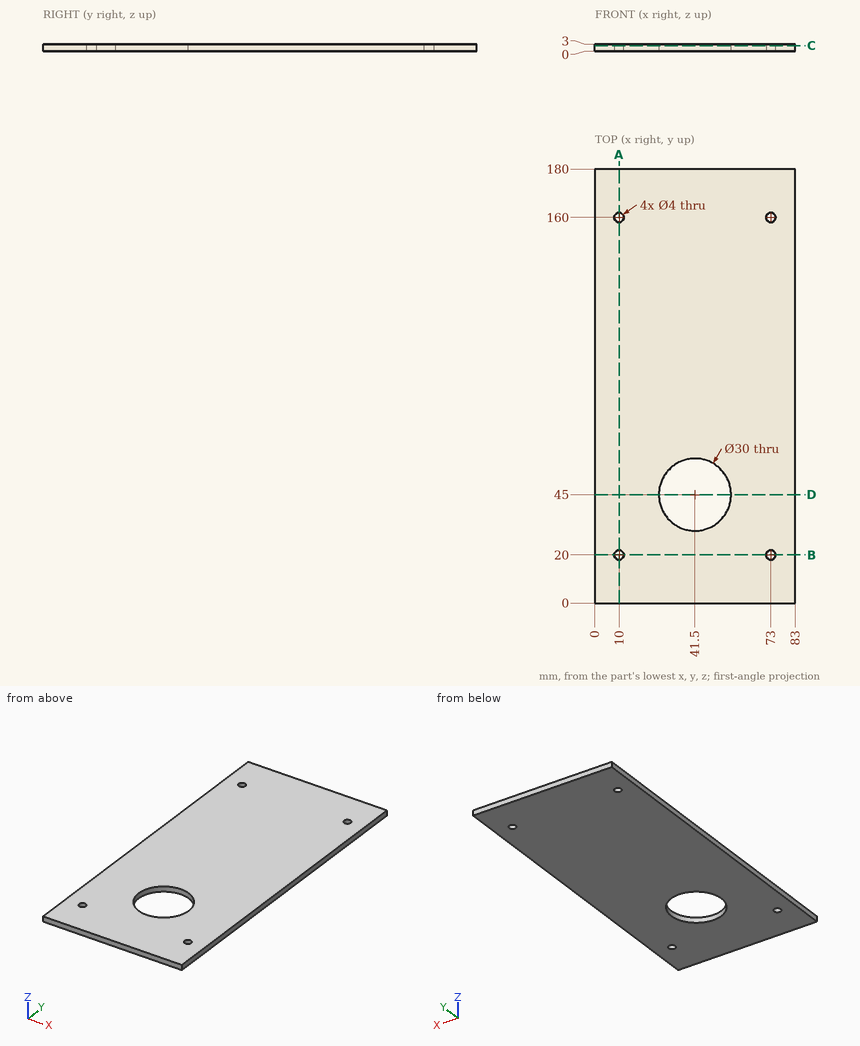
For this review, use the dimensioned drawing (mm, ordinates from the lowest corner) and the shaded views. Coordinates: 2 decimals unless noted, no trailing zeros. Loops run counter-clockwise (first coordinate to the right, second up) from the corner with the lowest first, then second, coordinate; pieces in that order, holes last. Notation, with made-up numbers: (35, 21) -> (80, 21) arc R26 ccw to (80, 50) -> close; hole circle Ø6 at (-24, 22). An arc over 180 degrees is marked (long way). Use a Markdown table: item, result. Add a question column.
1. Add section A-A on x = 10. Write out the cut boundary in (y, z).
2. Add section D-D on y = 45. Write out the cut boundary in (x, z).
3. Add section B-B on y = 20. Write out the cut boundary in (x, z), plus the area to 3 significant figures.
4. Add section C-C on z = 2.3. Write out the cut boundary in (x, y).
5. To check wall thickness, follow line 1 (X direction, y = 20, z = 0.8); line 2 (Y direction, x = 73, z = 2.1); line 3 (Y direction, x = 41.5, z = 0.85). State the ranges of each line that lie inside material, in increasing order.
Returned:
| question | item | result |
|---|---|---|
| 1 | outline | (0, 0) -> (18, 0) -> (18, 3) -> (0, 3) -> close; (22, 0) -> (158, 0) -> (158, 3) -> (22, 3) -> close; (162, 0) -> (180, 0) -> (180, 3) -> (162, 3) -> close |
| 2 | outline | (0, 0) -> (26.5, 0) -> (26.5, 3) -> (0, 3) -> close; (56.5, 0) -> (83, 0) -> (83, 3) -> (56.5, 3) -> close |
| 3 | outline | (0, 0) -> (8, 0) -> (8, 3) -> (0, 3) -> close; (12, 0) -> (71, 0) -> (71, 3) -> (12, 3) -> close; (75, 0) -> (83, 0) -> (83, 3) -> (75, 3) -> close |
| 3 | area | 225 mm² |
| 4 | outline | (0, 0) -> (83, 0) -> (83, 180) -> (0, 180) -> close; hole circle Ø4 at (10, 20); hole circle Ø4 at (10, 160); hole circle Ø30 at (41.5, 45); hole circle Ø4 at (73, 20); hole circle Ø4 at (73, 160) |
| 5 | line 1 | x = 0 to 8, 12 to 71, 75 to 83 |
| 5 | line 2 | y = 0 to 18, 22 to 158, 162 to 180 |
| 5 | line 3 | y = 0 to 30, 60 to 180 |
